Model file for the job. Use its own axes, mm. Coordinates: 2 decimals unless noted, no trailing zeros. Order: outer loops, then holes, each group sorted by start corner. A loop starts at its lowest first (then second) coordinate and runs counter-clockwise, first axis right, second up. Notation, with made-up numbers: (-4, 2) -> (1, 2) arc R18 ccw to (1, 17) -> close; hole circle Ø6 at (0, -29.5). An arc over 180 degrees is marked (long way). Return JSON: item names as keys, results as strings. Group by question number.
1) Cut at A-A (x = 263). Write the cut outline in (y, z), and give its area (3 significant figures).
2) Cut at C-C (z = 2.25). State how many separate pieces and enclosed holes the cut face has, and give its area (3 significant figures).
3) Cut at D-D (y = -176.5). Write the cut outline in (x, z), and give its area (3 significant figures).
4) Probe line 1 (Y direction, x = 263, z = 1.2); line 2 (X direction, y = -155, z = 2.25); line 3 (Y direction, x = 235, z = 2). List the from-to ranges inside material, lowest first.
5) Cut at B-B (y = -97.5). Write the cut outline in (x, z), and give its area (3 significant figures).
6) Flat gauge pins, fed straight in: pin 1 (3.5 mm diameter, centred on x = 235, y = -40, fed in from -Z); pin 2 (23 mm diameter, centred on x = 132.5, y = -97.5, fed in from -Z); pin 3 (1.5 mm diameter, centred on x = 149.5, z = 2, fed in from +Y); pin 4 (1.5 mm diameter, centred on x = 241.5, z = 0.5, fed in from +Y). Where does each tip first touch, or does it go through?
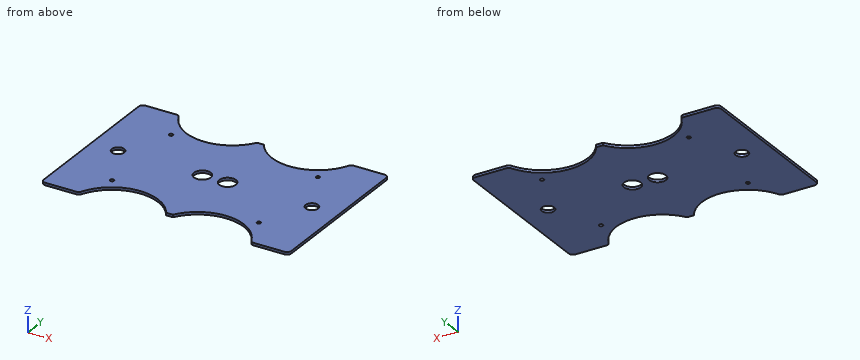
from build123d import *

# Parameters (mm, degrees)
ESQUISSE1_R        = 2.25
ESQUISSE1_R_2      = 7.5
ESQUISSE1_R_3      = 10
BOSS_EXTRU_1_DEPTH = 3


with BuildPart() as part:
    # Esquisse1 → Boss.-Extru.1 (new body)
    with BuildSketch(Plane.XY):
        with BuildLine():
            Line((5, 0), (41.684938398, 0))
            ThreePointArc((41.684938398, 0), (44.389031178, -0.794303597), (46.23397571, -2.924847105))
            ThreePointArc((46.23397571, -2.924847105), (93.045262331, -35.129096737), (143.5, -9))
            Line((143.5, -9), (151.5, -9))
            ThreePointArc((151.5, -9), (201.954737669, -35.129096737), (248.76602429, -2.924847105))
            ThreePointArc((248.76602429, -2.924847105), (250.610968822, -0.794303597), (253.315061602, 0))
            Line((253.315061602, 0), (290, 0))
            ThreePointArc((290, 0), (293.535533906, -1.464466094), (295, -5))
            Line((295, -5), (295, -190))
            ThreePointArc((295, -190), (293.535533906, -193.535533906), (290, -195))
            Line((290, -195), (253.315061602, -195))
            ThreePointArc((253.315061602, -195), (250.610968822, -194.205696403), (248.76602429, -192.075152895))
            ThreePointArc((248.76602429, -192.075152895), (201.954737669, -159.870903263), (151.5, -186))
            Line((151.5, -186), (143.5, -186))
            ThreePointArc((143.5, -186), (93.045262331, -159.870903263), (46.23397571, -192.075152895))
            ThreePointArc((46.23397571, -192.075152895), (44.389031178, -194.205696403), (41.684938398, -195))
            Line((41.684938398, -195), (5, -195))
            ThreePointArc((5, -195), (1.464466094, -193.535533906), (0, -190))
            Line((0, -190), (0, -5))
            ThreePointArc((0, -5), (1.464466094, -1.464466094), (5, 0))
        make_face()
        with Locations((60, -40)):
            Circle(ESQUISSE1_R, mode=Mode.SUBTRACT)
        with Locations((32, -97.5)):
            Circle(ESQUISSE1_R_2, mode=Mode.SUBTRACT)
        with Locations((263, -97.5)):
            Circle(ESQUISSE1_R_2, mode=Mode.SUBTRACT)
        with Locations((132.5, -97.5)):
            Circle(ESQUISSE1_R_3, mode=Mode.SUBTRACT)
        with Locations((162.5, -97.5)):
            Circle(ESQUISSE1_R_3, mode=Mode.SUBTRACT)
        with Locations((235, -40)):
            Circle(ESQUISSE1_R, mode=Mode.SUBTRACT)
        with Locations((235, -155)):
            Circle(ESQUISSE1_R, mode=Mode.SUBTRACT)
        with Locations((60, -155)):
            Circle(ESQUISSE1_R, mode=Mode.SUBTRACT)
    extrude(amount=BOSS_EXTRU_1_DEPTH)


solid = part.part
Answers below:
{
 "1": {"outline": "(-195, 0) -> (-105, 0) -> (-105, 3) -> (-195, 3) -> close; (-90, 0) -> (0, 0) -> (0, 3) -> (-90, 3) -> close", "area": "540 mm^2"},
 "2": {"separate pieces": "1", "enclosed holes": "8", "area": "45,900 mm^2"},
 "3": {"outline": "(0, 0) -> (56.88, 0) -> (56.88, 3) -> (0, 3) -> close; (136.1, 0) -> (158.9, 0) -> (158.9, 3) -> (136.1, 3) -> close; (238.12, 0) -> (295, 0) -> (295, 3) -> (238.12, 3) -> close", "area": "410 mm^2"},
 "4": {"line 1": "y = -195 to -105, -90 to 0", "line 2": "x = 0 to 57.75, 62.25 to 232.75, 237.25 to 295", "line 3": "y = -173.53 to -157.25, -152.75 to -42.25, -37.75 to -21.47"},
 "5": {"outline": "(0, 0) -> (24.5, 0) -> (24.5, 3) -> (0, 3) -> close; (39.5, 0) -> (122.5, 0) -> (122.5, 3) -> (39.5, 3) -> close; (142.5, 0) -> (152.5, 0) -> (152.5, 3) -> (142.5, 3) -> close; (172.5, 0) -> (255.5, 0) -> (255.5, 3) -> (172.5, 3) -> close; (270.5, 0) -> (295, 0) -> (295, 3) -> (270.5, 3) -> close", "area": "675 mm^2"},
 "6": {"pin 1": "passes through", "pin 2": "stops at z = 0", "pin 3": "stops at y = -9", "pin 4": "stops at y = -13.73"}
}
